Autodesk Inventor part; units mm, degrees
ref_plane "YZ Plane" through (0, 0, 0) normal (1, 0, 0) x (0, 1, 0)
ref_plane "XZ Plane" through (0, 0, 0) normal (0, 1, 0) x (-1, 0, 0)
ref_plane "XY Plane" through (0, 0, 0) normal (0, 0, 1) x (1, 0, 0)
sketch "Boceto1" plane through (0, 0, 0) normal (0, 0, 1) x (1, 0, 0)
  line L0 (-50, 0) -> (-50, -10)
  line L1 (-50, -10) -> (-45, -10)
  line L2 (-50, -10) -> (50, -10)
  line L3 (-45, -10) -> (-45, 0)
  line L4 (0, 0) -> (-50, 0)
  arc A0 (-45, 0) -> (-45, -10) centre (-45, -5) ccw
  line L5 (-50, -5) -> (-25, -5)
  line L6 (-25, -5) -> (-25, 25)
  line L7 (-25, 25) -> (-15, 25)
  line L8 (-15, 25) -> (-15, -5)
  line L9 (-15, -5) -> (-25, -5)
  line L10 (-20, 25) -> (-20, 5)
  line L11 (-22.5, 7.5) -> (-17.5, 7.5)
  line L12 (-17.5, 7.5) -> (-17.5, 22.5)
  line L13 (-17.5, 22.5) -> (-22.5, 22.5)
  line L14 (-22.5, 22.5) -> (-22.5, 7.5)
  line L15 (-22.5, 7.5) -> (-17.5, 22.5) construction
  line L16 (-17.5, 7.5) -> (-22.5, 22.5) construction
  line L17 (-22.5, 22.5) -> (-22.5, 21.5)
  line L18 (-22.5, 21.5) -> (-17.5, 21.5)
  line L19 (-22.5, 15) -> (-17.5, 15)
  arc A1 (-17.5, 21.5) -> (-22.5, 21.5) centre (-20, 18.875) ccw
  arc A2 (-22.5, 8.5) -> (-17.5, 8.5) centre (-20, 11.125) ccw
  line L20 (-25, -5) -> (-20, -5)
  line L21 (-20, -5) -> (-20, -10)
  line L22 (-20, -10) -> (-25, -10)
  line L23 (-25, -10) -> (-25, -5)
  line L24 (-25, 0) -> (-15, 0)
  line L25 (-15, -5) -> (-15, -10)
  point P0 (0, -10)
  point P1 (-20, 15)
  point P2 (-50, -5)
  point P3 (-20, 22.5)
  point P4 (-20, 7.5)
  point P5 (-22.5, 8.5)
  point P6 (-17.5, 8.5)
  point P7 (-20, -5)
  point P8 (-17.5, 8.5)
  point P9 (-22.5, 8.5)
  dimension "d0" = 5
  dimension "d1" = 25
  dimension "d2" = 30
  dimension "d3" = 10
  dimension "d4" = 20
  dimension "d5" = 5
  dimension "d6" = 15
  dimension "d7" = 1
extrude "Extrusión1" add sketch "Boceto1" against normal blind 5.5 contours L13 L12 A1 | A1 L14 L13 | L6 L7 L8 L4 | L4 L8 L9 L6 | L23 L9 L21 L2 | L21 L9 L25 L2 | A2 L12 L11 | L11 L14 A2
properties part number "PiezaAux"
Input: part model. Units: mm. Frame: model coordinates. A direction names the side the tool comes from. Round coordinates to 2 decimals unless told otherwise and drop trailing zeros. Loops run counter-clockwise (first coordinate to the right, second up) from the corner with the lowest first, then second, coordinate; pieces in that order, holes last. Notation, with made-up numbers: (40, 61) -> (46, 61) arc R37 ccw to (46, 99) -> close; hole circle Ø6 at (18, -12). An arc over 180 degrees is marked (long way). Use one line per item in the form item = value. Start each with the question number.
Item 1: Section query A-A on y = 18. Return the cut outline in (x, z), then the cut area to 3 significant figures.
Item 2: Set-up query: faces 4 (the face through (-25, 7, -3)), 5 (the face through (-20, 22.5, -2.7)). Return all of +Z, -Z, +X, -X, +Y, -Y with unobstructed straight access to the full face (end or side cutting, diameter ignored); none if empty.
Item 3: Section query B-B on z = -3.75. Return the cut outline in (x, y) (3 decimals), then the cut area to 3 significant figures.
Item 4: Mould query, pull axis X, two halves, no side actions, for faces 1 (the face through (-20, 4, 0)), 2 (the face through (-15, 8, -3)), 3 (the face through (-17.5, 15, -3)). Classes: pulls with the +X half, pulls with the -X half, needs draft (parallel to the pull), parting line crosses it, or undercut.
Item 5: Contact query for a flat-ended pin moving along its axis: pin 1 Ø1 at (x, y) = (-19, 21) entering from -Z. Output: stop coordinate, or through.
Item 6: Material intervals for L1, parallel to X at y = 19, z = -3.25; L2, parallel to Y at x = -21.5, z = -4.25; L3, parallel to Y at x = -19.5, z = -3.05, sorted ascending. Write a range as from..to.
Item 7: Section query C-C on x = -19.5. Return the cut outline in (y, z).
Ans:
q1.outline = (-25, -5.5) -> (-22.5, -5.5) -> (-22.5, 0) -> (-25, 0) -> close; (-17.5, -5.5) -> (-15, -5.5) -> (-15, 0) -> (-17.5, 0) -> close
q1.area = 27.5 mm^2
q2.face_4 = +Z, -Z, -X, +Y, -Y
q2.face_5 = +Z, -Z
q3.outline = (-25, -10) -> (-15, -10) -> (-15, 25) -> (-25, 25) -> close; hole (-22.5, 8.5) arc R3.625 ccw to (-17.5, 8.5) -> (-17.5, 21.5) arc R3.625 ccw to (-22.5, 21.5) -> close
q3.area = 278 mm^2
q4.face_1 = needs draft
q4.face_2 = pulls with the +X half
q4.face_3 = undercut
q5.pin_1 = through
q6.L1 = -25..-22.5, -17.5..-15
q6.L2 = -10..7.82, 22.18..25
q6.L3 = -10..7.53, 22.47..25
q7.outline = (-10, -5.5) -> (7.53, -5.5) -> (7.53, 0) -> (-10, 0) -> close; (22.47, -5.5) -> (25, -5.5) -> (25, 0) -> (22.47, 0) -> close
